Autodesk Inventor part; units mm, degrees
ref_plane "YZ Plane" through (0, 0, 0) normal (1, 0, 0) x (0, 1, 0)
ref_plane "XZ Plane" through (0, 0, 0) normal (0, 1, 0) x (-1, 0, 0)
ref_plane "XY Plane" through (0, 0, 0) normal (0, 0, 1) x (1, 0, 0)
sketch "Sketch1" plane through (0, 0, 0) normal (0, 0, 1) x (1, 0, 0)
  line L0 (0, 0) -> (25.4, 0)
  line L1 (25.4, 0) -> (25.4, 3.175)
  line L2 (3.175, 25.4) -> (0, 25.4)
  line L3 (0, 25.4) -> (0, 0)
  line L4 (3.175, 25.4) -> (3.175, 3.175)
  line L5 (3.175, 3.175) -> (25.4, 3.175)
  dimension "d0" = 25.4
  dimension "d1" = 25.4
  dimension "d2" = 3.175
  dimension "d3" = 3.175
extrude "Extrusion1" add sketch "Sketch1" along normal blind 152.4
sketch "Sketch3" plane through (0, 0, 0) normal (0, -1, 0) x (1, 0, 0)
  line L0 (25.4, 152.4) -> (0, 152.4)
  line L1 (0, 0) -> (0, 152.4)
  circle A0 centre (12.7, 107.95) radius 2.54
  circle A1 centre (12.7, 139.7) radius 2.54
  dimension "d20" = 12.7
  dimension "d21" = 31.75
  dimension "d22" = 5.08
  dimension "d23" = 12.7
extrude "Extrusion4" cut sketch "Sketch3" against normal blind 25.4
sketch "Sketch4" plane through (0, 0, 0) normal (-1, 0, 0) x (0, 0, 1)
  line L0 (0, 25.4) -> (0, 0)
  line L1 (0, 0) -> (152.4, 0)
  circle A0 centre (6.35, 19.05) radius 1.5875
  circle A1 centre (17.4625, 6.35) radius 1.5875
  line L2 (0, 25.4) -> (152.4, 25.4)
  line L3 (76.2, 25.4) -> (76.2, 0)
  circle A2 centre (146.05, 19.05) radius 1.5875
  circle A3 centre (134.9375, 6.35) radius 1.5875
  dimension "d26" = 6.35
  dimension "d27" = 19.05
  dimension "d28" = 3.175
  dimension "d29" = 6.35
  dimension "d30" = 17.4625
extrude "Extrusion5" cut sketch "Sketch4" against normal blind 25.4 contours A0 | A1 | A2 | A3
equation "\"d2\" = d3"
properties part number "8 ball corner L"
Input: part model. Units: mm. Frame: model coordinates. A direction names the side the tool comes from. Coordinates: 2 decimals unless noted, no trailing zeros. Loops run counter-clockwise (first coordinate to the right, second up) from the corner with the lowest first, then second, coordinate; pieces in that order, holes last. Notation, with made-up numbers: (57, -15) -> (115, -15) arc R15 ccw to (115, 0) -> close; hole circle Ø7 at (33.25, 46.5). An arc over 180 degrees is marked (long way). One line per item, written item: value.
(1) Cut plane D-D (z = 107.95). Output: boundary loops of the cut face in (x, y) (3 decimals).
Answer below:
outline: (0, 0) -> (10.16, 0) -> (10.16, 3.175) -> (3.175, 3.175) -> (3.175, 25.4) -> (0, 25.4) -> close; (15.24, 0) -> (25.4, 0) -> (25.4, 3.175) -> (15.24, 3.175) -> close
(2) Cut plane A-A (y = 19.05). Output: boundary loops of the cut face in (x, z) (1 decimal), then the cut area to 3 significant figures.
Answer below:
outline: (0, 0) -> (3.2, 0) -> (3.2, 4.8) -> (0, 4.8) -> close; (0, 7.9) -> (3.2, 7.9) -> (3.2, 144.5) -> (0, 144.5) -> close; (0, 147.6) -> (3.2, 147.6) -> (3.2, 152.4) -> (0, 152.4) -> close
area: 464 mm2
(3) Ray query, line 1 along Z through (x, y) = (12.7, 0.65); line 2 along Y through (x, z) = (0.75, 6.35); line 3 along X through (y, z) = (7, 99) (3 decimals). Return the intervals inside material, ascending.
Answer below:
line 1: z = 0 to 105.41, 110.49 to 137.16, 142.24 to 152.4
line 2: y = 0 to 17.46, 20.64 to 25.4
line 3: x = 0 to 3.175
(4) Cut plane C-C (x = 12.7). Output: boundary loops of the cut face in (y, z) (3 decimals).
Answer below:
outline: (0, 0) -> (3.175, 0) -> (3.175, 105.41) -> (0, 105.41) -> close; (0, 110.49) -> (3.175, 110.49) -> (3.175, 137.16) -> (0, 137.16) -> close; (0, 142.24) -> (3.175, 142.24) -> (3.175, 152.4) -> (0, 152.4) -> close
(5) Set-up query: faces 1 (the face through (0, 13, 75)), 2 (the face through (3.175, 14, 75)). Return all of +Z, -Z, +X, -X, +Y, -Y with unobstructed straight access to the full face (end or side cutting, diameter ignored); none if empty.
Answer below:
face 1: +Z, -Z, -X, +Y, -Y
face 2: +Z, -Z, +X, +Y
(6) Pin query (flat end, axial travel): pin 1 Ø6 at (x, z) = (12.7, 107.95) entering from -Y; pin 2 Ø8 at (y, z) = (12, 60) entering from +X (3 decimals); pin 3 Ø1 at (x, z) = (19.5, 35) entering from +Y (3 decimals). Return the tip coordinate at first contact, or that it passes through.
Answer below:
pin 1: stops at y = 0
pin 2: stops at x = 3.175
pin 3: stops at y = 3.175
(7) Cut plane B-B (z = 6.35). Output: boundary loops of the cut face in (x, y) (1 decimal), then the cut area to 3 significant figures.
Answer below:
outline: (0, 0) -> (25.4, 0) -> (25.4, 3.2) -> (3.2, 3.2) -> (3.2, 17.5) -> (0, 17.5) -> close; (0, 20.6) -> (3.2, 20.6) -> (3.2, 25.4) -> (0, 25.4) -> close
area: 141 mm2
(8) Draft query along X for faces 3 (the face through (12.15, 1.57, 105.47)), 4 (the face through (25.4, 2, 75)), 5 (the face through (1.565, 18.084, 144.79)), 6 (the face through (12.15, 1.57, 137.22)). Return one class per face: pulls with the +X half, pulls with the -X half, needs draft (parallel to the pull), parting line crosses it, or undercut.
Answer below:
face 3: undercut
face 4: pulls with the +X half
face 5: needs draft
face 6: undercut
